Can you work these out from the model? Positions are in its coordinate system, mm. Face numbers are marked on the shaded views. Give positions to 0.01 mm unless a question says otherwise; leave off trailing zeros. Write each loop counter-clockwise with the first axis right and the second up, starting at its lowest first coordinate (ties: lowest second). Pieces come first, ordered by that corner, then holes. Notation, with made-up numbers: M 11,-15 L 53,-15 A12 cw 53,-8 Z; hole C -14,16 d6. An arc over 180 degrees is marked long. Write each question's results on one line, items separated by ' | '.
from build123d import *

# Parameters (mm, degrees)
ESQUISSE1_R        = 7.5
ESQUISSE1_R_2      = 1.5
BOSS_EXTRU_1_DEPTH = 3


with BuildPart() as part:
    # Esquisse1 → Boss.-Extru.1 (new body)
    with BuildSketch(Plane(origin=(0, 0, 0), x_dir=(1, 0, 0), z_dir=(0, 1, 0))):
        Circle(ESQUISSE1_R)
        with Locations((-3.5, 0)):
            Circle(ESQUISSE1_R_2, mode=Mode.SUBTRACT)
        with Locations((3.5, 0)):
            Circle(ESQUISSE1_R_2, mode=Mode.SUBTRACT)
        with BuildLine():
            ThreePointArc((1.991071429, 2.878477821), (0.25, 0), (1.991071429, -2.878477821))
            ThreePointArc((1.991071429, -2.878477821), (0, -3.5), (-1.991071429, -2.878477821))
            ThreePointArc((-1.991071429, -2.878477821), (-0.25, 0), (-1.991071429, 2.878477821))
            ThreePointArc((-1.991071429, 2.878477821), (0, 3.5), (1.991071429, 2.878477821))
        make_face(mode=Mode.SUBTRACT)
    extrude(amount=BOSS_EXTRU_1_DEPTH)


solid = part.part
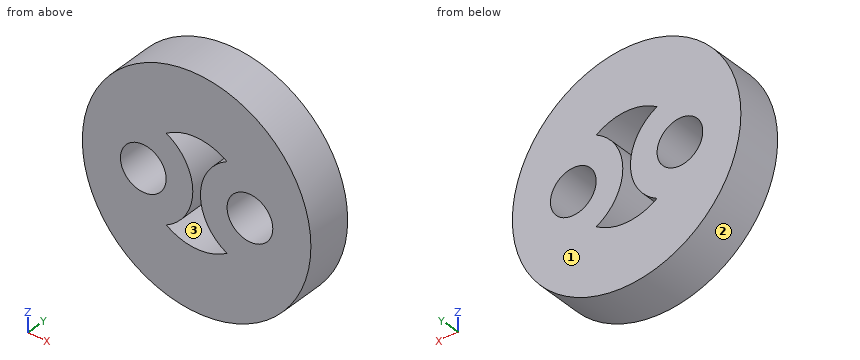
Item 1: I'm going to push a flat-ended pin straight in: pin 1 (2.5 mm diameter, centred on x = 3.5, z = 0, fed in from -Y). Where does the tip first touch, or does it pass through?
Geometry says:
pin 1: passes through
Item 2: I want a section at C-C, the plane y = 1.55. Please give me the cut outline in (x, z).
Geometry says:
outline: C 0,0 d15; hole C -3.5,0 d3; hole M -1.99,-2.88 A3.5 ccw 1.99,-2.88 A3.25 cw 1.99,2.88 A3.5 ccw -1.99,2.88 A3.25 cw Z; hole C 3.5,0 d3
Item 3: I want a section at D-D, the plane z = 2.25. Please give me the cut outline in (x, y), and give its area (3 significant figures).
Geometry says:
outline: M -7.15,0 L -1.15,0 L -1.15,3 L -7.15,3 Z; M 1.15,0 L 7.15,0 L 7.15,3 L 1.15,3 Z | area: 36.0 mm2
Item 4: If I drill on line 1 (X direction, y = 0.9, z = 0); line 2 (Z direction, x = 0.5, y = 2.1); line 3 (Z direction, x = -1, y = 1.7), over which ranges is the centre line in solid material (lowest first)? Write a range as from..to.
Geometry says:
line 1: x = -7.5..-5, -2..-0.25, 0.25..2, 5..7.5 | line 2: z = -7.48..-3.46, -1.25..1.25, 3.46..7.48 | line 3: z = -7.43..-3.35, -2.08..2.08, 3.35..7.43
Item 5: I want a section at A-A, the plane x = 0. Please give me the cut outline in (y, z).
Geometry says:
outline: M 0,-7.5 L 3,-7.5 L 3,-3.5 L 0,-3.5 Z; M 0,3.5 L 3,3.5 L 3,7.5 L 0,7.5 Z
Item 6: I want a section at B-B, the plane z = 0. Please give me the cut outline in (x, y).
Geometry says:
outline: M -7.5,0 L -5,0 L -5,3 L -7.5,3 Z; M -2,0 L -0.25,0 L -0.25,3 L -2,3 Z; M 0.25,0 L 2,0 L 2,3 L 0.25,3 Z; M 5,0 L 7.5,0 L 7.5,3 L 5,3 Z
Item 7: Thinking about a two-plate mould opening in Z: for the marked faces 1, 2 and 3, which applies, +Z half, -Z half, draft (parallel to the pull), parting line (faces both ways), or undercut?
Geometry says:
face 1: draft | face 2: parting line | face 3: undercut
